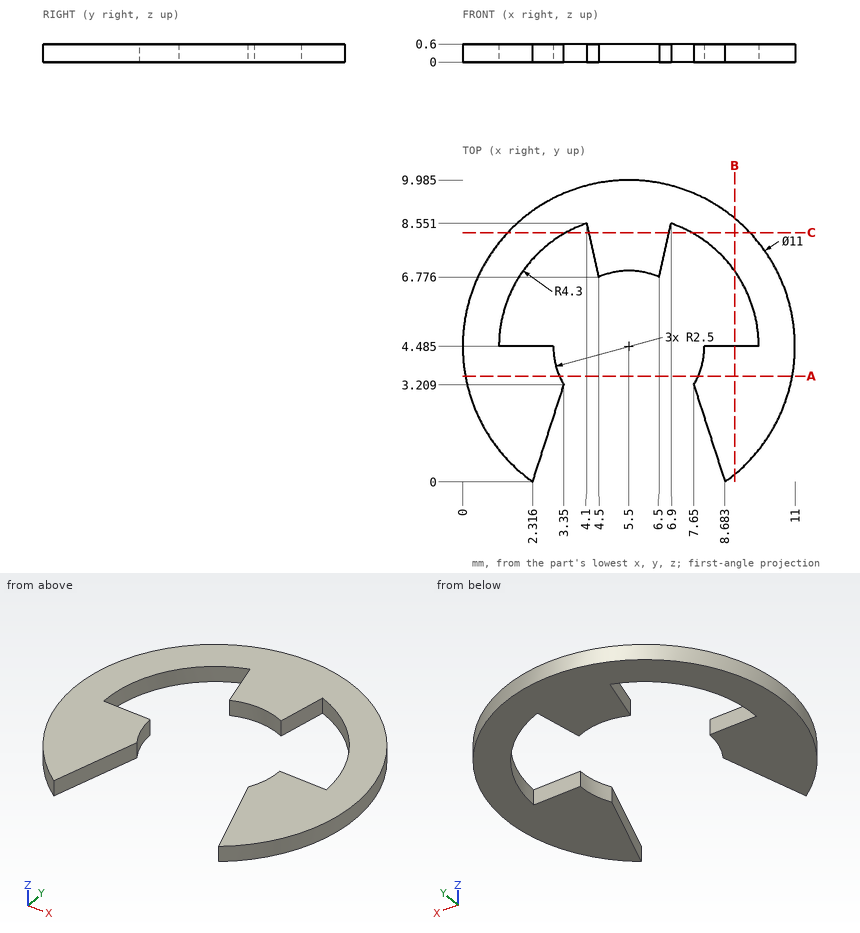
The drawing under review shows one solid part. Ordinate dimensions are in mm from its lowest x, y, z. Give positions to 0.01 mm unless a question says otherwise; leave off trailing zeros. Write each loop counter-clockwise with the first axis right and the second up, starting at its lowest first coordinate (ties: lowest second). Pieces come first, ordered by that corner, then holes. Notation, with made-up numbers: (74.25, -18) -> (105.25, -18) arc R20 ccw to (105.25, 18) -> close; hole circle Ø9 at (-14.75, -37). An arc over 180 degrees is marked (long way). Answer in a Markdown table with one row per item.
(1) To check wall thickness, follow probe 1 along X at (y, z) = (2.5, 0.35); probe 2 along X at (y, z) = (4.25, 0.35) (1 decimal); probe 3 along Y at (x, z) = (2, 0.45) (1 decimal). State the ranges of each line that lie inside material, in increasing order.
Results:
| item | result |
|---|---|
| probe 1 | 0.37 to 3.12, 7.88 to 10.63 |
| probe 2 | 0 to 3, 8 to 11 |
| probe 3 | 0.2 to 4.5, 7 to 8.7 |
(2) Consider section C-C (y = 8.25). State the section outline as (x, z) points.
Results:
| item | result |
|---|---|
| outline | (1.49, 0) -> (3.42, 0) -> (3.42, 0.6) -> (1.49, 0.6) -> close; (4.17, 0) -> (6.83, 0) -> (6.83, 0.6) -> (4.17, 0.6) -> close; (7.58, 0) -> (9.51, 0) -> (9.51, 0.6) -> (7.58, 0.6) -> close |
(3) Consider section A-A (y = 3.5). State the section outline as (x, z) points.
Results:
| item | result |
|---|---|
| outline | (0.09, 0) -> (3.2, 0) -> (3.2, 0.6) -> (0.09, 0.6) -> close; (7.8, 0) -> (10.91, 0) -> (10.91, 0.6) -> (7.8, 0.6) -> close |
(4) Consider section B-B (x = 9). State the section outline as (y, z) points (1 decimal).
Results:
| item | result |
|---|---|
| outline | (0.2, 0) -> (4.5, 0) -> (4.5, 0.6) -> (0.2, 0.6) -> close; (7, 0) -> (8.7, 0) -> (8.7, 0.6) -> (7, 0.6) -> close |
